```python
from build123d import *

# Parameters (mm, degrees)
TOP_BLADE_PROFILE_R     = 1.1
BASIC_BLADE_SHAPE_DEPTH = 0.9
EDGE_GRIND_SIZE         = 0.072
EDGE_GRIND_SIZE2        = 0.098954535
BLADE_ROOT_FILLET_R     = 3
BLADE_END_FILLET_R      = 3


with BuildPart() as part:
    # top blade profile → basic blade shape (new body)
    with BuildSketch(Plane.XY):
        with BuildLine():
            Line((-14.743176388, 14.743176388), (-20.043176388, 14.743176388))
            ThreePointArc((-20.043176388, 14.743176388), (-33.304536559, -7.535711071), (-34.497327018, -33.435320159))
            Line((-34.497327018, -33.435320159), (-26.655881065, -31.850477781))
            ThreePointArc((-26.655881065, -31.850477781), (-24.405908014, -20.396982829), (-17.885844028, -10.715366695))
            ThreePointArc((-17.885844028, -10.715366695), (-11.75653181, -17.219362932), (-3.467222551, -20.559690362))
            ThreePointArc((-3.467222551, -20.559690362), (20.559690362, -3.467222551), (3.467222551, 20.559690362))
            ThreePointArc((3.467222551, 20.559690362), (-6.343874402, 19.861464135), (-14.743176388, 14.743176388))
        make_face()
        with Locations((-17.5, 0)):
            Circle(TOP_BLADE_PROFILE_R, mode=Mode.SUBTRACT)
        with Locations((0, -17.5)):
            Circle(TOP_BLADE_PROFILE_R, mode=Mode.SUBTRACT)
        with Locations((17.5, 0)):
            Circle(TOP_BLADE_PROFILE_R, mode=Mode.SUBTRACT)
        with Locations((0, 17.5)):
            Circle(TOP_BLADE_PROFILE_R, mode=Mode.SUBTRACT)
        with BuildLine():
            Line((-15.713707666, 6.258524906), (-14.021091263, 5.041725875))
            ThreePointArc((-14.021091263, 5.041725875), (-14.333173834, 4.07064219), (-14.578087267, 3.080482372))
            ThreePointArc((-14.578087267, 3.080482372), (-13.45, 0), (-14.578087267, -3.080482372))
            ThreePointArc((-14.578087267, -3.080482372), (-10.53589104, -10.53589104), (-3.080482372, -14.578087267))
            ThreePointArc((-3.080482372, -14.578087267), (0, -13.45), (3.080482372, -14.578087267))
            ThreePointArc((3.080482372, -14.578087267), (10.53589104, -10.53589104), (14.578087267, -3.080482372))
            ThreePointArc((14.578087267, -3.080482372), (13.45, 0), (14.578087267, 3.080482372))
            ThreePointArc((14.578087267, 3.080482372), (10.53589104, 10.53589104), (3.080482372, 14.578087267))
            ThreePointArc((3.080482372, 14.578087267), (0, 13.45), (-3.080482372, 14.578087267))
            ThreePointArc((-3.080482372, 14.578087267), (-8.250663905, 12.407116713), (-12.252281094, 8.478891908))
            Line((-12.252281094, 8.478891908), (-14.32615504, 9.092015713))
            ThreePointArc((-14.32615504, 9.092015713), (-16.216729433, 8.261339025), (-15.713707666, 6.258524906))
        make_face(mode=Mode.SUBTRACT)
    extrude(amount=BASIC_BLADE_SHAPE_DEPTH)

    # blade grind: sweep along a path in grind path
    with BuildLine(Plane.XY.offset(0.9)) as blade_grind_path:
        ThreePointArc((-14.282047318, 19.76313332), (-32.075420619, -3.915533869), (-34.497327018, -33.435320159))
    # Sketch1 → blade grind (sweep, cut)
    with BuildSketch(Plane(origin=(5.138564907, -25.424470933, 0), x_dir=(0.9801807441283484, 0.19810529735470822, 0), z_dir=(0.19810529735470822, -0.9801807441283484, 0))):
        Polygon((-40.43732971, 0), (-40.43732971, 0.8), (-37.23732971, 0), align=None)
    sweep(path=blade_grind_path.line, mode=Mode.SUBTRACT)

    # edge grind
    edge_grind_edges = [part.edges().sort_by_distance(p)[0] for p in [
        (-33.304536559, -7.535711071, 0.8),
    ]]
    edge_grind_side = [part.faces().sort_by_distance(p)[0] for p in [
        (-31.257621093, -6.37778083, 0.4),
    ]]
    chamfer(edge_grind_edges, length=EDGE_GRIND_SIZE, length2=EDGE_GRIND_SIZE2, reference=edge_grind_side[0])

    # blade root fillet
    blade_root_fillet_edges = [part.edges().sort_by_distance(p)[0] for p in [
        (-17.885844028, -10.715366695, 0.45),
    ]]
    fillet(blade_root_fillet_edges, radius=BLADE_ROOT_FILLET_R)

    # blade end fillet
    blade_end_fillet_edges = [part.edges().sort_by_distance(p)[0] for p in [
        (-26.655881065, -31.850477781, 0.45),
    ]]
    fillet(blade_end_fillet_edges, radius=BLADE_END_FILLET_R)


solid = part.part
```
Geometry: final body of the model. Coordinates: model frame, mm. A direction names the side the tool comes from. Coordinates: 2 decimals unless noted, no trailing zeros. Loops run counter-clockwise (first coordinate to the right, second up) from the corner with the lowest first, then second, coordinate; pieces in that order, holes last. Notation, with made-up numbers: M 80,-34.75 L 95,-34.75 A19 cw 95,-28.75 Z; hole C 28.5,44.5 d10. An arc over 180 degrees is marked long. Put each result on its own line as item: value.
(1) Cut plane A-A on x = 0. Return the cut outline in (y, z).
Answer sheet:
outline: M -20.85,0 L -18.6,0 L -18.6,0.9 L -20.85,0.9 Z; M -16.4,0 L -13.45,0 L -13.45,0.9 L -16.4,0.9 Z; M 13.45,0 L 16.4,0 L 16.4,0.9 L 13.45,0.9 Z; M 18.6,0 L 20.85,0 L 20.85,0.9 L 18.6,0.9 Z
(2) Cut plane B-B on x = -9. Return the cut outline in (y, z), then the cut area to 3 significant figures.
Answer sheet:
outline: M -18.81,0 L -11.87,0 L -11.87,0.9 L -18.81,0.9 Z; M 11.87,0 L 18.81,0 L 18.81,0.9 L 11.87,0.9 Z
area: 12.5 mm^2
(3) First-contact query: pin 1 (0.5 mm diameter, centred on x = -16.5, z = 0.5, fed in from +Y). Flat tip, straight axial feed; report the tip coordinate or a pass-through.
Answer sheet:
pin 1: stops at y = 14.74
(4) Access query for faces 4 (the face through (-27.303, -31.34, 0.456)), 5 (the face through (10.62, 10.45, 0.44)). Directions: +Z, -Z, +X, -X, +Y, -Y. A direction counts if a zero-diameter tool reaches every point of the face in a straight line with its end or side. Return the directions, or none.
Answer sheet:
face 4: +Z, -Z, +X, -Y
face 5: +Z, -Z
(5) Draft query along Y for faces 1 (the face through (-14, -6, 0)), 2 (the face through (-24.76, -21.29, 0.44)), 3 (the face through (-0.238, 16.426, 0.444)). Return one class per face: pulls with the +Y half, pulls with the -Y half, needs draft (parallel to the pull), parting line crosses it, or undercut.
Answer sheet:
face 1: needs draft
face 2: pulls with the -Y half
face 3: undercut
(6) Material intervals for probe 1 along Y at (x, z) = (0, 0.45); probe 2 along Y at (x, z) = (-16.5, 0.25); probe 3 along Y at (x, z) = (17.5, 0.55), sorted ascending.
Answer sheet:
probe 1: y = -20.85 to -18.6, -16.4 to -13.45, 13.45 to 16.4, 18.6 to 20.85
probe 2: y = -12.98 to -0.46, 0.46 to 14.74
probe 3: y = -11.33 to -1.1, 1.1 to 11.33
(7) Cut plane C-C on y = -17.5. State how many separate pieces and enclosed holes the cut face has, then the cut area to 3 significant figures.
Answer sheet:
separate pieces: 3
enclosed holes: 0
area: 28.2 mm^2
